Can you work these out from the model? Positions are in its coordinate system, mm. Coordinates: 2 decimals unless noted, no trailing zeros. Write each loop counter-clockwise with the first axis right and the second up, starting at its lowest first coordinate (ties: lowest second). Pieces come first, ordered by that corner, then holes. Notation, with made-up numbers: (-26, 34.25) -> (15, 34.25) arc R16 ccw to (15, 51.25) -> close; hole circle Ø8 at (87.25, 82.5). An arc over 180 degrees is marked (long way). Answer as CSV lines item,"result". Start each with the question number.
Autodesk Inventor part; units mm, degrees
ref_plane "YZ Plane" through (0, 0, 0) normal (1, 0, 0) x (0, 1, 0)
ref_plane "XZ Plane" through (0, 0, 0) normal (0, 1, 0) x (-1, 0, 0)
ref_plane "XY Plane" through (0, 0, 0) normal (0, 0, 1) x (1, 0, 0)
sketch "Sketch1" plane through (0, 0, 0) normal (0, 0, 1) x (1, 0, 0)
  line L0 (0, 0) -> (22.5, 0)
  line L1 (22.5, 0) -> (22.5, 3)
  line L2 (22.5, 3) -> (0, 3)
  line L3 (0, 3) -> (0, 0)
  dimension "d0" = 22.5
  dimension "d1" = 3
extrude "Extrusion1" add sketch "Sketch1" along normal blind 86.75
sketch "Sketch2" plane through (0, 3, 0) normal (0, 1, 0) x (1, 0, 0)
  line L0 (0, 0) -> (22.5, 0)
  line L1 (11.25, 0) -> (11.25, -2)
  line L2 (11.25, 0) -> (13.25, 0) construction
  line L3 (11.25, -2) -> (4.75, -2)
  line L4 (4.75, -2) -> (4.75, -7.5)
  line L5 (4.75, -7.5) -> (11.25, -7.5)
  line L6 (11.25, -7.5) -> (11.25, -2)
  line L7 (11.25, -2) -> (17.75, -2)
  line L8 (17.75, -2) -> (17.75, -7.5)
  line L9 (17.75, -7.5) -> (11.25, -7.5)
  line L10 (11.25, -7.5) -> (11.25, -2)
  dimension "d4" = 2
  dimension "d5" = 90
  dimension "d6" = 6.5
  dimension "d7" = 5.5
  dimension "d8" = 6.5
  dimension "d9" = 5.5
extrude "Extrusion2" cut sketch "Sketch2" against normal blind 3
sketch "Sketch3" plane through (0, 3, 0) normal (0, 1, 0) x (1, 0, 0)
  line L0 (4.75, -7.5) -> (17.75, -7.5)
  line L1 (11.25, -7.5) -> (11.25, -10)
  line L2 (11.25, -7.5) -> (13.75, -7.5) construction
  line L3 (11.25, -10) -> (7.25, -10)
  line L4 (7.25, -10) -> (7.25, -13)
  line L5 (7.25, -13) -> (11.25, -13)
  line L6 (11.25, -13) -> (11.25, -10)
  line L7 (11.25, -10) -> (15.25, -10)
  line L8 (15.25, -10) -> (15.25, -13)
  line L9 (15.25, -13) -> (11.25, -13)
  line L10 (11.25, -13) -> (11.25, -10)
  point P0 (0, 0)
  dimension "d12" = 2.5
  dimension "d13" = 90
  dimension "d14" = 4
  dimension "d15" = 3
  dimension "d16" = 4
  dimension "d17" = 3
extrude "Extrusion3" cut sketch "Sketch3" against normal blind 3
sketch "Sketch4" plane through (0, 3, 0) normal (0, 1, 0) x (1, 0, 0)
  point P0 (0, 0)
chamfer "Chamfer1" distance 1.5 angle 45 4 edges at (22.5, 3, 43.375) (11.25, 3, 86.75) (0, 3, 43.375) (11.25, 3, 0)
chamfer "Chamfer2" distance 1 angle 45 4 edges at (0, 0.75, 86.75) (22.5, 0.75, 86.75) (22.5, 0.75, 0) (0, 0.75, 0)
chamfer "Chamfer3" distance 0.8165 angle 45 4 edges at (1, 2.5, 1) (21.5, 2.5, 1) (1, 2.5, 85.75) (21.5, 2.5, 85.75)
sketch "Sketch5" plane through (22.5, 0, 85.75) normal (1, 0, 0) x (0, 0, -1)
  line L0 (83.25, 3) -> (84.75, 1.5)
  line L1 (84.75, 1.5) -> (0, 1.5)
  line L2 (0, 1.5) -> (0, 3)
  line L3 (0, 3) -> (84.75, 3)
  line L4 (84.75, 3) -> (84.75, 1.5)
  point P0 (85.75, 0)
  dimension "d29" = 84.75
  dimension "d30" = 1.5
extrude "Extrusion4" add sketch "Sketch5" against normal blind 2.5
sketch "Sketch6" plane through (22.5, 0, 85.75) normal (1, 0, 0) x (0, 0, -1)
  line L0 (0, 3) -> (84.75, 3)
  line L1 (0, 3) -> (84.75, 3)
  line L2 (84.75, 3) -> (84.75, 2)
  line L3 (84.75, 2) -> (0, 2)
  line L4 (0, 2) -> (0, 3)
  point P0 (85.75, 0)
  dimension "d33" = 84.75
  dimension "d34" = 1
extrude "Extrusion5" add sketch "Sketch6" along normal blind 1
sketch "Sketch7" plane through (0, 0, 1) normal (-1, 0, 0) x (0, 0, 1)
  line L0 (0, 1.5) -> (1.5, 3)
  line L1 (0, 1.5) -> (84.75, 1.5)
  line L2 (84.75, 1.5) -> (84.75, 3)
  line L3 (84.75, 3) -> (0, 3)
  line L4 (0, 3) -> (0, 1.5)
  point P0 (-1, 0)
  dimension "d37" = 84.75
  dimension "d38" = 1.5
extrude "Extrusion6" add sketch "Sketch7" against normal blind 2.5
sketch "Sketch8" plane through (0, 0, 1) normal (-1, 0, 0) x (0, 0, 1)
  line L0 (0, 3) -> (0.5, 3)
  line L1 (0, 2) -> (84.75, 2)
  line L2 (0, 3) -> (84.75, 3)
  line L3 (84.75, 3) -> (84.75, 2)
  line L4 (84.75, 2) -> (0, 2)
  line L5 (0, 2) -> (0, 3)
  point P0 (-1, 0)
  dimension "d41" = 84.75
  dimension "d42" = 1
extrude "Extrusion7" add sketch "Sketch8" along normal blind 1
chamfer "Chamfer4" distance 0.5 angle 45 8 edges at (21.75, 3, 85.75) (23, 2, 85.75) (0.75, 3, 85.75) (-0.5, 2, 85.75) (0.75, 3, 1) (-0.5, 2, 1) (21.75, 3, 1) (23, 2, 1)
properties part number "Battery-Management-Case-Cover"
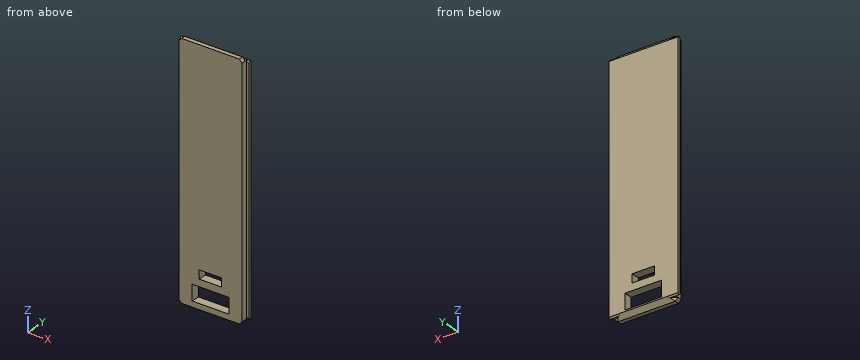
Q1. Imagine slicing it at C-C (z = 50). Write out the boundary of the cut face in (x, y).
Q2. I need wall thicknesses on L1, parallel to Z at x = 12.5, y = 0.7; L2, parallel to Z at x = 17.25, y = 0.9; L3, parallel to Z at x = 11.25, y = 2. Which ranges of each line are inside material? Lowest first, please.
Q3. Imagine slicing it at B-B (y = 0.55). Write out the boundary of the cut face in (x, z).
Q4. Imagine slicing it at A-A (x = 16.75). Write out the boundary of the cut face in (y, z).
Q5. For pin 1 (1.5 mm diameter, centred on y = 0.5, z = 52, fed in from -X); pin 2 (0.6 mm diameter, centred on y = 3, z = 1, fed in from -X); pin 3 (0.8 mm diameter, centred on x = -0.5, z = 64.5, fed in from -Y); pin 4 (0.9 mm diameter, centred on y = 1.5, z = 3.5, fed in from +X), each with a flat end and sliding along its axis, tell me the tip position at first contact or that it passes through.
Entries:
1,outline,"(-1, 2) -> (0, 2) -> (0, 0) -> (22.5, 0) -> (22.5, 2) -> (23.5, 2) -> (23.5, 3) -> (-1, 3) -> close"
2,L1,"0 to 2, 7.5 to 10, 13 to 86.75"
2,L2,"0 to 2, 7.5 to 86.75"
2,L3,"0.5 to 2, 7.5 to 10, 13 to 86.25"
3,outline,"(0, 1) -> (1, 0) -> (21.5, 0) -> (22.5, 1) -> (22.5, 85.75) -> (21.5, 86.75) -> (1, 86.75) -> (0, 85.75) -> close; hole (4.75, 2) -> (17.75, 2) -> (17.75, 7.5) -> (4.75, 7.5) -> close; hole (7.25, 10) -> (15.25, 10) -> (15.25, 13) -> (7.25, 13) -> close"
4,outline,"(0, 0) -> (1.5, 0) -> (3, 1.5) -> (3, 2) -> (0, 2) -> close; (0, 7.5) -> (3, 7.5) -> (3, 85.25) -> (1.5, 86.75) -> (0, 86.75) -> close"
5,pin 1,"x = 0"
5,pin 2,"through"
5,pin 3,"y = 2"
5,pin 4,"x = 22.5"
